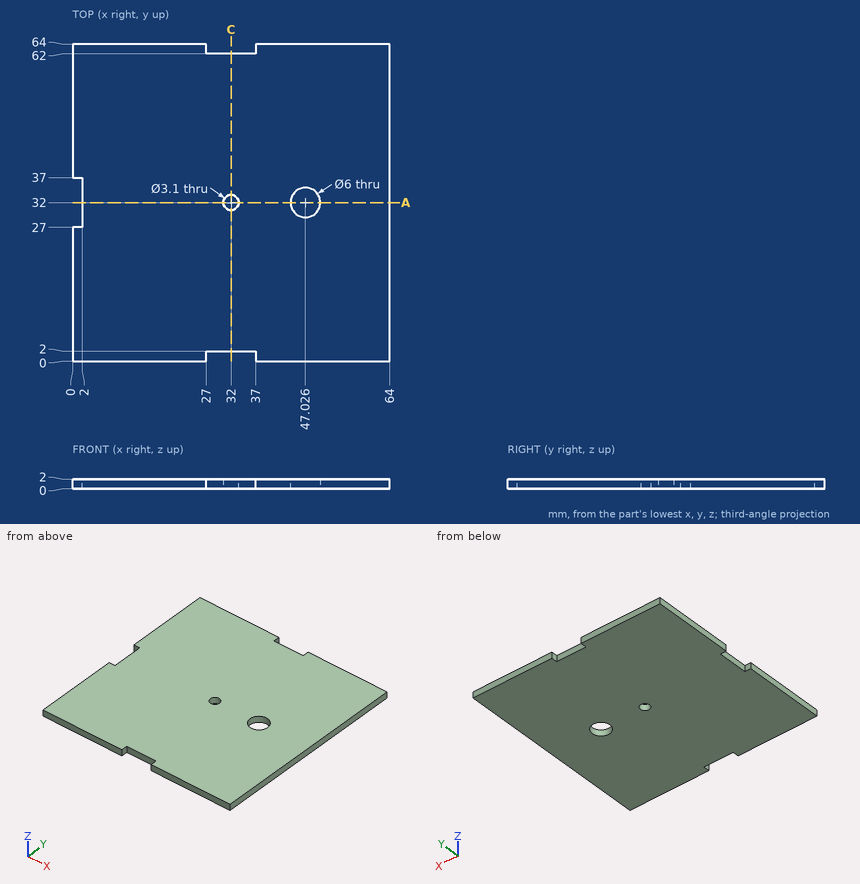
Design review of the part shown in the three views and the two pictorial views. Dimensions are in mm from the part's minimum x, y and z. Round coordinates to 2 decimals unless told otherwise and drop trailing zeros. Write each loop counter-clockwise with the first axis right and the second up, starting at its lowest first coordinate (ties: lowest second). Pieces come first, ordered by that corner, then holes. Notation, with made-up numbers: M -11,-25 L 40,-25 A32 ccw 40,2 Z; hole C 48.25,-35.75 d5. An arc over 180 degrees is marked long. Use a Markdown table: item, result. Add a question column.
Q1. We need section C-C, the plane x = 32. State the section outline as (y, z) points, plus the area to 3 significant figures.
Q2. To check wall thickness, follow line 1 (Y direction, x = 32, z = 1.05); line 2 (Y direction, x = 33, z = 0.25) (1 decimal); line 3 (Y direction, x = 34.5, z = 1.8). State the ranges of each line that lie inside material, in increasing order.
Q3. We need section A-A, the plane y = 32. Count the separate pieces of the cut face and the enclosed holes in it, plus the area to 3 significant figures.
Q4. Insertion check: pin 1 (5 mm diameter, centred on x = 47.03, y = 32, fed in from +Z); pin 2 (0.6 mm diameter, centred on y = 33.5, z = 1.5, fed in from -X); pin 3 (1 mm diameter, centred on x = 32, z = 1.5, fed in from +Y). Each pin has a flat end and moves straight along its axis. Give the tip position at first contact, or say it passes through.
Findings below:
| question | item | result |
|---|---|---|
| 1 | outline | M 2,0 L 30.45,0 L 30.45,2 L 2,2 Z; M 33.55,0 L 62,0 L 62,2 L 33.55,2 Z |
| 1 | area | 114 mm² |
| 2 | line 1 | y = 2 to 30.45, 33.55 to 62 |
| 2 | line 2 | y = 2 to 30.8, 33.2 to 62 |
| 2 | line 3 | y = 2 to 62 |
| 3 | separate pieces | 3 |
| 3 | enclosed holes | 0 |
| 3 | area | 106 mm² |
| 4 | pin 1 | passes through |
| 4 | pin 2 | stops at x = 2 |
| 4 | pin 3 | stops at y = 62 |
